For this review, use the dimensioned drawing (mm, ordinates from the lowest corner) and the shaded views. Round coordinates to 2 decimals unless told otherwise and drop trailing zeros. Write each loop counter-clockwise with the first axis right and the second up, starting at its lowest first coordinate (ties: lowest second). Pieces come first, ordered by that corner, then holes. Notation, with made-up numbers: (-0.5, 38.25) - (22.5, 38.25) arc R13 cw to (22.5, 52.25) - close; hole circle Ø4 at (10, 4.25). An arc over 180 degrees is marked (long way). Return JSON: item names as keys, results as strings.
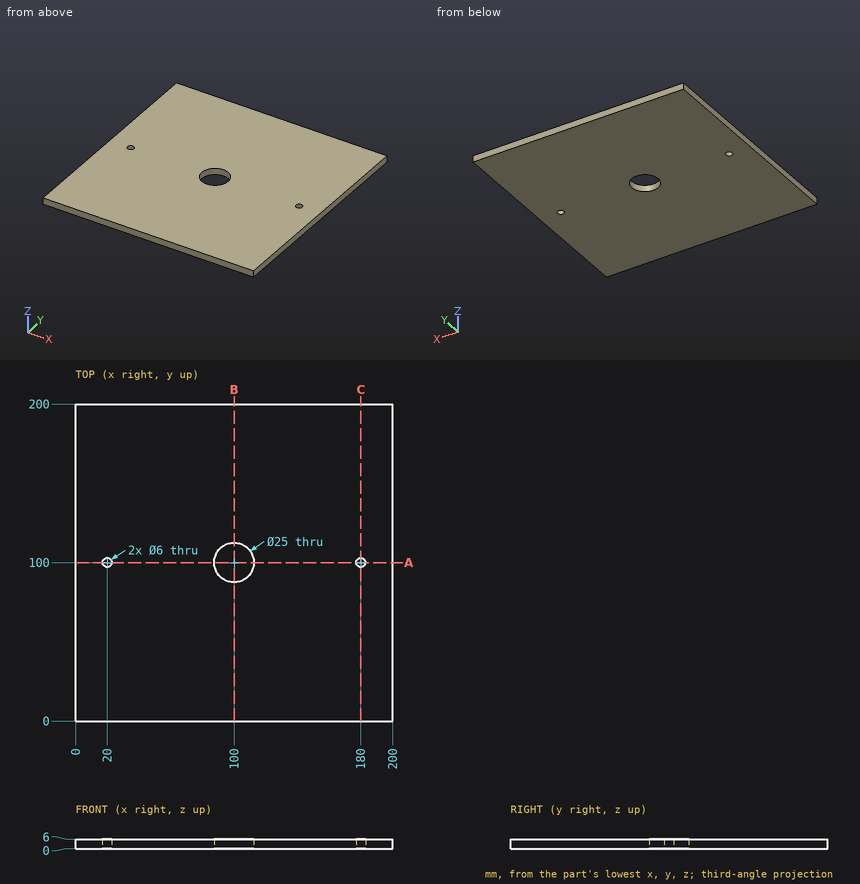
(1) Wall thickness on line 1 (Y direction, x = 180, z = 2.6); line 2 (Y direction, x = 100, z = 2.25): over which ranges is each line inside the solid? List them lowest first.
Filled in:
{"line 1": "y = 0 to 97, 103 to 200", "line 2": "y = 0 to 87.5, 112.5 to 200"}
(2) Add section C-C (x = 180). Write out the cut boundary in (y, z).
Filled in:
{"outline": "(0, 0) - (97, 0) - (97, 6) - (0, 6) - close; (103, 0) - (200, 0) - (200, 6) - (103, 6) - close"}
(3) Clearance check with flat-ended pins moving along their axes: pin 1 Ø2 at (x, y) = (55.5, 159) entering from -Z; pin 2 Ø6 at (x, y) = (99, 108.5) entering from +Z (3 decimals). State where each tip first meets the part, or that it passes through.
Filled in:
{"pin 1": "stops at z = 0", "pin 2": "passes through"}
(4) Add section A-A (y = 100). Write out the cut boundary in (x, z).
Filled in:
{"outline": "(0, 0) - (17, 0) - (17, 6) - (0, 6) - close; (23, 0) - (87.5, 0) - (87.5, 6) - (23, 6) - close; (112.5, 0) - (177, 0) - (177, 6) - (112.5, 6) - close; (183, 0) - (200, 0) - (200, 6) - (183, 6) - close"}
(5) Add section B-B (x = 100). Write out the cut boundary in (y, z).
Filled in:
{"outline": "(0, 0) - (87.5, 0) - (87.5, 6) - (0, 6) - close; (112.5, 0) - (200, 0) - (200, 6) - (112.5, 6) - close"}
